```python
from build123d import *

# Parameters (mm, degrees)
SKETCH1_W                                        = 44.45
SKETCH1_H                                        = 60.96
BOSS_EXTRUDE1_DEPTH                              = 7.9375
CBORE_FOR_1_4_SOCKET_HEAD_CAP_SCREW1_D           = 6.7564
CBORE_FOR_1_4_SOCKET_HEAD_CAP_SCREW1_CBORE_D     = 11.1125
CBORE_FOR_1_4_SOCKET_HEAD_CAP_SCREW1_CBORE_DEPTH = 6.35
SKETCH4_W                                        = 7.62
SKETCH4_H                                        = 27.94
CUT_EXTRUDE1_DEPTH                               = 45.45
F_8_32_TAPPED_HOLE1_D                            = 3.4544


with BuildPart() as part:
    # Sketch1 → Boss-Extrude1 (new body, symmetric)
    with BuildSketch(Plane.XY):
        Rectangle(SKETCH1_W, SKETCH1_H)
    extrude(amount=BOSS_EXTRUDE1_DEPTH, both=True)

    # CBORE for 1/4 Socket Head Cap Screw1 (through all)
    with Locations(Plane.XY.offset(7.9375)):
        with Locations((-12.7, -3.81), (12.7, -3.81), (12.7, -22.86), (-12.7, -22.86)):
            CounterBoreHole(CBORE_FOR_1_4_SOCKET_HEAD_CAP_SCREW1_D / 2, CBORE_FOR_1_4_SOCKET_HEAD_CAP_SCREW1_CBORE_D / 2, CBORE_FOR_1_4_SOCKET_HEAD_CAP_SCREW1_CBORE_DEPTH)

    # Sketch4 → Cut-Extrude1 (cut, through all)
    with BuildSketch(Plane(origin=(22.225, 0, 0), x_dir=(0, 0, -1), z_dir=(1, 0, 0))):
        with Locations((4.1275, 16.51)):
            Rectangle(SKETCH4_W, SKETCH4_H)
    extrude(amount=-CUT_EXTRUDE1_DEPTH, mode=Mode.SUBTRACT)

    # #8-32 Tapped Hole1 (through all)
    with Locations(Plane.XY.offset(7.9375)):
        with Locations((-11.43, 19.939), (11.43, 19.939)):
            Hole(F_8_32_TAPPED_HOLE1_D / 2)


solid = part.part
```
CAD build for the part. Positions are in the model's coordinates, mm. A direction names the side the tool comes from. Give positions to 0.01 mm unless a question says otherwise; leave off trailing zeros. Order: outer loops, then holes, each group sorted by start corner. A loop starts at its lowest first (then second) coordinate and runs counter-clockwise, first axis right, second up.
(1) Saw through at C-C, the plane z = -4.25. Give the cut face in (x, y) (3 decimals).
(2) Flat gauge pins, fed straight in: pin 1 (1 mm diameter, centred on y = 5, z = -6, fed in from -X); pin 2 (8 mm diameter, centred on x = -10.5, z = -5.5, fed in from +Y). Where does each tip first touch, or does it go through?
(3) Saw through at B-B, the plane x = 11.43. Give the cut face in (y, z), then the cut area to 3 significant figures.
(4) Saw through at A-A, the plane y = -3.81. Give the cut face in (x, z) (1 decimal), then the cut area to 3 significant figures.
(5) Tool access for faces 1 (the flat face through (0, -30.48, 0)), 2 (the flat face through (-12.8, -26.5, 1.588)): list every direction of +Z, -Z, +X, -X, +Y, -Y with a clear straight run to the whole face (end or side of a thin tool).
(6) Saw through at D-D, the plane z = 0.75. Give the cut face in (x, y) (3 decimals), then the cut area to 3 significant figures.
(7) Drill centre lines: L1, parallel to Y at x = -12.7, z = -5; L2, parallel to Y at x = -11.43, z = 6; L3, parallel to Y at x = 12, z = 7. Where is each one in solid material? Low to high.
(8) Mould opens along X. For faces 3 (the flat face through (22.225, -7, 2)), 4 (the cylindrical face through (-17.1, -7.2, 4.8)), 5 (the flat face through (0, 2.54, -4)), 6 (the flat face through (-22.225, -7, 2)) say: released by +X, released by -X, zero draft, split by the parting line, or undercut.
Results found:
1. outline: (-22.225, -30.48) - (22.225, -30.48) - (22.225, 2.54) - (-22.225, 2.54) - close; hole circle Ø6.756 at (-12.7, -22.86); hole circle Ø6.756 at (-12.7, -3.81); hole circle Ø6.756 at (12.7, -22.86); hole circle Ø6.756 at (12.7, -3.81)
2. pin 1: passes through
2. pin 2: stops at y = 2.54
3. outline: (-30.48, -7.94) - (-25.99, -7.94) - (-25.99, 1.59) - (-28.27, 1.59) - (-28.27, 7.94) - (-30.48, 7.94) - close; (-19.73, -7.94) - (-6.94, -7.94) - (-6.94, 1.59) - (-9.22, 1.59) - (-9.22, 7.94) - (-17.45, 7.94) - (-17.45, 1.59) - (-19.73, 1.59) - close; (-0.68, -7.94) - (2.54, -7.94) - (2.54, -0.32) - (18.21, -0.32) - (18.21, 7.94) - (1.6, 7.94) - (1.6, 1.59) - (-0.68, 1.59) - close; (21.67, -0.32) - (30.48, -0.32) - (30.48, 7.94) - (21.67, 7.94) - close
3. area: 470 mm2
4. outline: (-22.2, -7.9) - (-16.1, -7.9) - (-16.1, 1.6) - (-18.3, 1.6) - (-18.3, 7.9) - (-22.2, 7.9) - close; (-9.3, -7.9) - (9.3, -7.9) - (9.3, 1.6) - (7.1, 1.6) - (7.1, 7.9) - (-7.1, 7.9) - (-7.1, 1.6) - (-9.3, 1.6) - close; (16.1, -7.9) - (22.2, -7.9) - (22.2, 7.9) - (18.3, 7.9) - (18.3, 1.6) - (16.1, 1.6) - close
4. area: 436 mm2
5. face 1: +Z, -Z, +X, -X, -Y
5. face 2: +Z
6. outline: (-22.225, -30.48) - (22.225, -30.48) - (22.225, 30.48) - (-22.225, 30.48) - close; hole circle Ø6.756 at (-12.7, -22.86); hole circle Ø6.756 at (-12.7, -3.81); hole circle Ø3.454 at (-11.43, 19.939); hole circle Ø6.756 at (12.7, -22.86); hole circle Ø6.756 at (12.7, -3.81); hole circle Ø3.454 at (11.43, 19.939)
6. area: 2,550 mm2
7. L1: y = -30.48 to -26.24, -19.48 to -7.19, -0.43 to 2.54
7. L2: y = -30.48 to -28.27, -17.45 to -9.22, 1.6 to 18.21, 21.67 to 30.48
7. L3: y = -30.48 to -28.37, -17.35 to -9.32, 1.7 to 18.31, 21.57 to 30.48
8. face 3: released by +X
8. face 4: undercut
8. face 5: zero draft
8. face 6: released by -X
